Could you check a few things on this model? Use its own coordinates, in mm. Round coordinates to 2 decimals unless told otherwise and drop trailing zeros. Loops run counter-clockwise (first coordinate to the right, second up) from the corner with the lowest first, then second, coordinate; pieces in that order, holes last. Notation, with made-up numbers: (72.25, -15) -> (96.25, -15) arc R12 cw to (96.25, -2) -> close; hole circle Ø1 at (-39.5, -32.5). An arc over 180 degrees is marked (long way). Write each question's results on one line, items separated by ' | '.
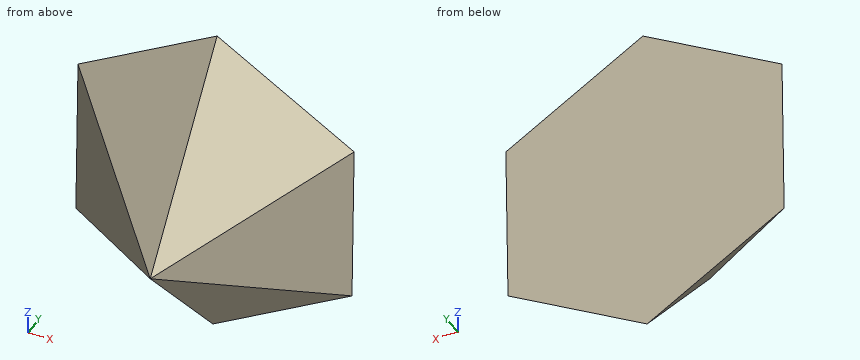
from build123d import *


with BuildPart() as f3:
    # F0 (on Front) → F3 section 0
    with BuildSketch(Plane.XZ, mode=Mode.PRIVATE) as f3_s0:
        Polygon((1.213273, 91.136256), (-78.319676, 46.618853), (-79.532949, -44.517403), (-1.213273, -91.136256), (78.319676, -46.618853), (79.532949, 44.517403), align=None)
    loft([f3_s0.sketch, Vertex(14.658035, -100, 7.94503)])


solid = f3.part
1) I want a section at C-C, the plane x = 7. Write out the boundary of the cut face in (y, z).
Model answer:
outline: (-91.87, 3.68) -> (-51.75, -39.86) -> (0, -86.54) -> (0, 87.69) -> (-43.04, 55.33) -> (-91.76, 11.13) -> close
2) I want a section at D-D, the plane z = -74.5. Write out the boundary of the cut face in (x, y), plus the area to 3 significant figures.
Model answer:
outline: (-29.16, 0) -> (1.45, -16.79) -> (28.51, 0) -> close | area: 484 mm2
3) I want a section at B-B, the plane z = -36.5. Write out the boundary of the cut face in (x, y).
Model answer:
outline: (-79.43, 0) -> (-65.14, -15.28) -> (7.54, -55.14) -> (66.51, -18.54) -> (78.45, 0) -> close
4) I need wall thicknesses on line 1 (Z direction, x = 50, y = -37); line 2 (X direction, y = -11, z = -28.5); line 3 (Z direction, x = -45.5, y = -7). Which ranges of each line are inside material? Lowest first, please.
Model answer:
line 1: z = -29.1 to 34.28 | line 2: x = -69.04 to 71.48 | line 3: z = -57.18 to 58.64
5) I'm going to push flat-ended pins straight in: pin 1 (1 mm diameter, centred on x = 2, z = -14, fed in from -Y); pin 2 (1 mm diameter, centred on x = -52, y = -20.5, fed in from -Z); pin 3 (8 mm diameter, centred on x = 14.5, y = -23, fed in from -Z). Where does each tip first touch, or does it pass through?
Model answer:
pin 1: stops at y = -73.37 | pin 2: stops at z = -39.28 | pin 3: stops at z = -65.84
6) I want a section at A-A, the plane y = -43.5. Write out the boundary of the cut face in (x, z).
Model answer:
outline: (-38.56, -21.7) -> (5.69, -48.04) -> (50.63, -22.88) -> (51.31, 28.61) -> (7.06, 54.95) -> (-37.87, 29.8) -> close
